Work out the finished part from the listing and answer in its coordinate system (mm). Face numbers are marked on the shaded views. A direction names the side the tool comes from. Coordinates: 2 decimals unless noted, no trailing zeros. Order: outer loops, then holes, each group sorted by start corner. A loop starts at its lowest first (then second) coordinate and runs counter-clockwise, first axis right, second up. Notation, with made-up numbers: M -32.75,56.25 L -27.75,56.25 A31 cw -27.75,88.25 Z; hole C 26.5,68.5 d10. An arc over 180 degrees is marked long. Use a Markdown table: item, result.
from build123d import *

# Parameters (mm, degrees)
F1_DEPTH     = 63.5
F0_W         = 25.4
F0_H         = 19.05
F2_DEPTH     = 25.4
F3_DEPTH     = 7.9375
F5_R         = 6.35
F6_R         = 5.08
F7_T1_DEPTH  = 69.85
F7_T3_DEPTH  = 49.2125
F7_T5_DEPTH  = 31.75
F7_T8_ANGLE  = 90
F7_T10_ANGLE = 90
F8_R         = 5.08


# Not quite as in the source:
# - a fillet or chamfer that OpenCascade refuses, or shapes differently, is made with other operations: its cross-section is extruded or revolved along the edge and cut away or added


with BuildPart() as f1:
    # F0 (on Front) → F1 (new body, symmetric)
    with BuildSketch(Plane.XZ):
        Polygon((22.225, 9.525), (-41.275, 9.525), (-41.275, -9.525), (41.275, -9.525), (41.275, 9.525), align=None)
    extrude(amount=F1_DEPTH, both=True)

    # F0 (on Front) → F2 (join, symmetric)
    with BuildSketch(Plane.XZ):
        with BuildLine():
            Line((22.225, 27.0002), (22.225, 9.525))
            Line((22.225, 9.525), (41.275, 9.525))
            Line((41.275, 9.525), (41.275, 27.0002))
            ThreePointArc((41.275, 27.0002), (45.9246798487, 38.2255201513), (57.15, 42.8752))
            Line((57.15, 42.8752), (60.325, 42.8752))
            Line((60.325, 42.8752), (60.325, 61.9252))
            Line((60.325, 61.9252), (57.15, 61.9252))
            add(Edge.make_bspline(
                [(56.0885572702, 61.9090665575), (56.4433633619, 61.9154910812), (56.7971916203, 61.9208676872), (57.15, 61.9252)],
                knots=[110.5707934898, 110.5707934898, 110.5707934898, 110.5707934898, 111.5045361635, 111.5045361635, 111.5045361635, 111.5045361635], degree=3))
            ThreePointArc((56.0885572702, 61.9090665575), (32.0818278255, 51.3177321287), (22.225, 27.0002))
        make_face()
        with Locations((73.025, 52.4002)):
            Rectangle(F0_W, F0_H)
    extrude(amount=F2_DEPTH, both=True)

    # F0 (on Front) → F3 (join, symmetric)
    with BuildSketch(Plane.XZ):
        with BuildLine():
            add(Edge.make_bspline(
                [(-41.275, 9.525), (-41.6531258736, 45.6930648181), (14.073565129, 61.1482951996), (56.0885572702, 61.9090665575)],
                knots=[0, 0, 0, 0, 110.5707934898, 110.5707934898, 110.5707934898, 110.5707934898], degree=3))
            Line((-41.275, 9.525), (22.225, 9.525))
            Line((22.225, 9.525), (22.225, 27.0002))
            ThreePointArc((22.225, 27.0002), (32.0818278255, 51.3177321287), (56.0885572702, 61.9090665575))
        make_face()
    extrude(amount=F3_DEPTH, both=True)

    # F0 (on Front) → F4 (revolve)
    with BuildSketch(Plane.XZ):
        Polygon((85.725, 66.675), (85.725, 61.9252), (85.725, 42.8752), (85.725, 38.1), (111.125, 38.1), (111.125, 66.675), align=None)
    revolve(axis=Axis((85.725, 0, 52.3875), (0, 0, 1)))

    # F5
    f5_edges = [f1.edges().sort_by_distance(p)[0] for p in [
        (-41.275, -63.5, 0),
        (41.275, -63.5, 0),
        (41.275, 63.5, 0),
        (-41.275, 63.5, 0),
    ]]
    fillet(f5_edges, radius=F5_R)

    # F6
    f6_edges = [f1.edges().sort_by_distance(p)[0] for p in [
        (0, -63.5, -9.525),
    ]]
    fillet(f6_edges, radius=F6_R)

    # F7: fillet of radius 5.08 on 1 edges, made by hand

    # F7_s2 → F7_t1 (cut)
    with BuildSketch(Plane.YZ.offset(-34.925)):
        with BuildLine():
            ThreePointArc((58.42, 9.525), (62.0121024484, 8.0371024484), (63.5, 4.445))
            Line((63.5, 4.445), (63.5, 9.525))
            Line((63.5, 9.525), (58.42, 9.525))
        make_face()
    extrude(amount=F7_T1_DEPTH, mode=Mode.SUBTRACT)

    # F7_s4 → F7_t3 (cut)
    with BuildSketch(Plane.XZ.offset(-57.15)):
        with BuildLine():
            ThreePointArc((-36.195, 9.525), (-39.7871024484, 8.0371024484), (-41.275, 4.445))
            Line((-41.275, 4.445), (-41.275, 9.525))
            Line((-41.275, 9.525), (-36.195, 9.525))
        make_face()
    extrude(amount=F7_T3_DEPTH, mode=Mode.SUBTRACT)

    # F7_s6 → F7_t5 (cut)
    with BuildSketch(Plane.XZ.offset(-57.15)):
        with BuildLine():
            ThreePointArc((41.275, 4.445), (39.7871024484, 8.0371024484), (36.195, 9.525))
            Line((36.195, 9.525), (41.275, 9.525))
            Line((41.275, 9.525), (41.275, 4.445))
        make_face()
    extrude(amount=F7_T5_DEPTH, mode=Mode.SUBTRACT)

    # F7_s7 → F7_t8 (revolve, cut)
    with BuildSketch(Plane.XZ.offset(-57.15)):
        with BuildLine():
            ThreePointArc((41.275, 4.445), (39.7871024484, 8.0371024484), (36.195, 9.525))
            Line((36.195, 9.525), (41.275, 9.525))
            Line((41.275, 9.525), (41.275, 4.445))
        make_face()
    revolve(axis=Axis((34.925, 57.15, 9.525), (0, 0, 1)), revolution_arc=F7_T8_ANGLE, mode=Mode.SUBTRACT)

    # F7_s9 → F7_t10 (revolve, cut)
    with BuildSketch(Plane.XZ.offset(-57.15)):
        with BuildLine():
            ThreePointArc((-36.195, 9.525), (-39.7871024484, 8.0371024484), (-41.275, 4.445))
            Line((-41.275, 4.445), (-41.275, 9.525))
            Line((-41.275, 9.525), (-36.195, 9.525))
        make_face()
    revolve(axis=Axis((-34.925, 57.15, 9.525), (0, 0, -1)), revolution_arc=F7_T10_ANGLE, mode=Mode.SUBTRACT)

    # F8
    f8_edges = [f1.edges().sort_by_distance(p)[0] for p in [
        (0, -63.5, 9.525),
        (41.275, -41.275, 9.525),
        (39.415128, -61.640128, 9.525),
        (-39.415128, -61.640128, 9.525),
        (-41.275, -32.54375, 9.525),
    ]]
    fillet(f8_edges, radius=F8_R)


solid = f1.part
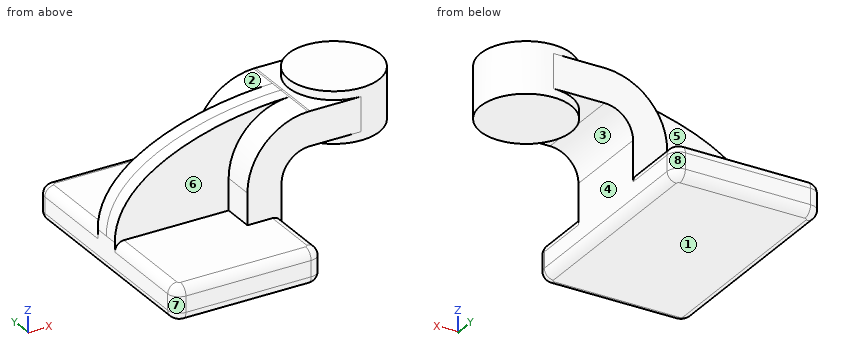
1. For a pull along X with two mould halves and no side action, classify the marked faces 1, 2 and 3 as +X half, -X half, draft (parallel to the pull), parting line (faces both ways), or undercut.
Answers below:
| item | result |
|---|---|
| face 1 | draft |
| face 2 | -X half |
| face 3 | undercut |
2. Flat-ended cylindrical pins translate along their axes: P1, Ø8.5, axis at x = 65, y = -6, coming from the -Z side; P2, Ø12, axis at x = 57.5, z = 39.5, coming from the -Y side; P3, Ø9.5, axis at y = 15, z = 6.5, coming from the +X side (3 decimals); P4, Ø1, axis at x = 17.5, z = 58.5, coming from the +Y side. Find the tip coordinate at first contact, or state that the pin passes through.
Answers below:
| item | result |
|---|---|
| P1 | z = 38.1 |
| P2 | y = -25.4 |
| P3 | x = 41.275 |
| P4 | through |
3. Section A-A on z = 1.5 is taken. Determine the outline of the cut face in (x, y) (3 decimals).
Answers below:
| item | result |
|---|---|
| outline | M -41.275,-57.15 A6.35 ccw -34.925,-63.5 L 34.925,-63.5 A6.35 ccw 41.275,-57.15 L 41.275,57.15 A6.35 ccw 34.925,63.5 L -34.925,63.5 A6.35 ccw -41.275,57.15 Z |
4. Find the intervals of material crossed by probe 1 along X at (y, z) = (-19.5, 11) (3 decimals); probe 2 along Z at (x, y) = (59.5, 18); probe 3 along Z at (x, y) = (4, -48) (3 decimals), in increasing order.
Answers below:
| item | result |
|---|---|
| probe 1 | 22.225 to 41.275 |
| probe 2 | 42.88 to 61.93 |
| probe 3 | -9.525 to 9.525 |
5. Section B-B on y = 49.5 is taken. Determine the outline of the cut face in (x, z) (3 decimals), then the cut area to 3 significant figures.
Answers below:
| item | result |
|---|---|
| outline | M -41.275,-4.445 A5.08 ccw -36.195,-9.525 L 36.195,-9.525 A5.08 ccw 41.275,-4.445 L 41.275,4.445 A5.08 ccw 36.195,9.525 L -36.195,9.525 A5.08 ccw -41.275,4.445 Z |
| area | 1,550 mm² |
6. For the marked faces 4, 5, 6, 7 and 8, determine the directions among +Z, -Z, +X, -X, +Y, -Y from which every point of the face is accessible in a straight line to the end or side of a thin tool.
Answers below:
| item | result |
|---|---|
| face 4 | -Z, +X, +Y, -Y |
| face 5 | +Z, -X, +Y |
| face 6 | +Z, -X, -Y |
| face 7 | +Z, -Z, -X, -Y |
| face 8 | +Z, -Z, +X, +Y |
